Model file for the job. Use its own axes, mm. A direction names the side the tool comes from. Coordinates: 2 decimals unless noted, no trailing zeros. Write each loop counter-clockwise with the first axis right and the second up, starting at its lowest first coordinate (ties: lowest second). Pieces come first, ordered by that corner, then holes. Notation, with made-up numbers: (-11.75, -2.75) - (26.25, -2.75) arc R4 ccw to (26.25, 1.25) - close; hole circle Ø10 at (56.25, 54). An arc over 180 degrees is marked (long way). Put each result on its own line as item: value. Start each with the question number.
1. Saw through at C-C, the plane z = 0. Write the cut outline in (x, y).
2. Which spindle directions (+Z, -Z, +X, -X, +Y, -Y) get a long thin tool onto all of the face, cutting with end or side? Do faces 4 (the face through (25.19, -0.49, -25.72)), 5 (the face through (-25.19, -0.49, 25.72)), 6 (the face through (-27.15, 3.01, 20.35)). Say none if no direction does.
3. Saw through at B-B, the plane x = 0. Write the cut outline in (y, z), plus the area to 3 significant figures.
4. Pull direction Z, two halves, no side cores. Call faces 1 (the face through (27.44, 5.4, 19.86)), 2 (the face through (-1.5, -1, 35)), 3 (the face through (35, -1, -1.5)): released by +Z, released by -Z, zero draft, split by the parting line, or undercut.
5. Saw through at A-A, the plane y = 5. Write the cut outline in (x, z).
6. Drop flat-ended pins along their axis: P1, Ø1, axis at y = 3.5, z = -33, coming from the -X side; P2, Ø1.5, axis at x = -31, y = 5, coming from the +Z side; P3, Ø4, axis at x = -27, z = -6.5, coming from the +Y side. Give the stop position or say it passes through.
7. Drill centre lines: L1, parallel to X at y = -1.25, z = 6.5; L2, parallel to Y at x = -10, z = 29; L3, parallel to Z at x = -2, y = 2.5. Where is each one in solid material? Low to high. Write a range as from..to.
```python
from build123d import *

# Parameters (mm, degrees)
SKETCH1_R           = 40
BOSS_EXTRUDE1_DEPTH = 2
SKETCH2_W           = 8.4
SKETCH2_H           = 2.75
BOSS_EXTRUDE2_DEPTH = 4
SKETCH3_R           = 36
SKETCH3_R_2         = 34
BOSS_EXTRUDE3_DEPTH = 2
FILLET2_R           = 1
CUT_EXTRUDE1_DEPTH  = 2
SKETCH5_W           = 8.4
SKETCH5_H           = 2.75
SKETCH5_W_2         = 8.1
SKETCH5_H_2         = 2.45
CUT_EXTRUDE2_DEPTH  = 4
FILLET3_R           = 2


with BuildPart() as part:
    # Sketch1 → Boss-Extrude1 (new body)
    with BuildSketch(Plane(origin=(0, 0, 0), x_dir=(1, 0, 0), z_dir=(0, 1, 0))):
        with Locations(Location((0, 0, 0), (0, 0, 270))):
            Circle(SKETCH1_R)
    extrude(amount=BOSS_EXTRUDE1_DEPTH)

    # Sketch2 → Boss-Extrude2 (add)
    with BuildSketch(Plane(origin=(0, 2, 0), x_dir=(1, 0, 0), z_dir=(0, 1, 0))):
        with Locations((0, 33.675)):
            Rectangle(SKETCH2_W, SKETCH2_H)
        Polygon((32.454190403, -13.887693304), (28.254190403, -21.162306696), (25.872620542, -19.787306696), (30.072620542, -12.512693304), align=None)
        Polygon((-28.254190403, -21.162306696), (-32.454190403, -13.887693304), (-30.072620542, -12.512693304), (-25.872620542, -19.787306696), align=None)
    extrude(amount=BOSS_EXTRUDE2_DEPTH)

    # Sketch3 → Boss-Extrude3 (add)
    with BuildSketch(Plane.XZ):
        with Locations(Location((0, 0, 0), (0, 0, 90))):
            Circle(SKETCH3_R)
        with Locations(Location((0, 0, 0), (0, 0, 270))):
            Circle(SKETCH3_R_2, mode=Mode.SUBTRACT)
    extrude(amount=BOSS_EXTRUDE3_DEPTH)

    # Fillet2
    fillet2_edges = [part.edges().sort_by_distance(p)[0] for p in [
        (0, -2, -36),
        (0, -2, 34),
    ]]
    fillet(fillet2_edges, radius=FILLET2_R - 0.0001)  # a hair under: the kernel refuses the full size

    # Sketch4 → Cut-Extrude1 (cut)
    with BuildSketch(Plane.XZ):
        Polygon((-1.5, -40), (-1.5, -1.5), (-40, -1.5), (-40, 1.5), (-1.5, 1.5), (-1.5, 40), (1.5, 40), (1.5, 1.5), (40, 1.5), (40, -1.5), (1.5, -1.5), (1.5, -40), align=None)
    extrude(amount=CUT_EXTRUDE1_DEPTH, mode=Mode.SUBTRACT)

    # Sketch5 → Cut-Extrude2 (cut)
    # profile 1 of 3: a face of its own
    with BuildSketch(Plane(origin=(0, 6, 0), x_dir=(1, 0, 0), z_dir=(0, 1, 0))):
        Polygon((32.454190403, -13.887693304), (30.072620542, -12.512693304), (25.872620542, -19.787306696), (28.254190403, -21.162306696), align=None)
        Polygon((32.249286592, -13.942597115), (30.127524353, -12.717597115), (26.077524353, -19.732402885), (28.199286592, -20.957402885), align=None, mode=Mode.SUBTRACT)
    # profile 2 of 3: a face of its own
    with BuildSketch(Plane(origin=(0, 6, 0), x_dir=(1, 0, 0), z_dir=(0, 1, 0))):
        Polygon((-28.254190403, -21.162306696), (-25.872620542, -19.787306696), (-30.072620542, -12.512693304), (-32.454190403, -13.887693304), align=None)
        Polygon((-28.199286592, -20.957402885), (-26.077524353, -19.732402885), (-30.127524353, -12.717597115), (-32.249286592, -13.942597115), align=None, mode=Mode.SUBTRACT)
    # profile 3 of 3: a face of its own
    with BuildSketch(Plane(origin=(0, 6, 0), x_dir=(1, 0, 0), z_dir=(0, 1, 0))):
        with Locations((0, 33.675)):
            Rectangle(SKETCH5_W, SKETCH5_H)
        with Locations((0, 33.675)):
            Rectangle(SKETCH5_W_2, SKETCH5_H_2, mode=Mode.SUBTRACT)
    extrude(amount=-CUT_EXTRUDE2_DEPTH, mode=Mode.SUBTRACT)

    # Fillet3
    fillet3_edges = [part.edges().sort_by_distance(p)[0] for p in [
        (31.188405472, 6, 13.330097115),
        (27.138405472, 6, 20.344902885),
        (-27.138405472, 6, 20.344902885),
        (-31.188405472, 6, 13.330097115),
        (-4.05, 6, -33.675),
        (4.05, 6, -33.675),
    ]]
    fillet(fillet3_edges, radius=FILLET3_R)


solid = part.part
```
Final values:
1. outline: (-40, 0) - (40, 0) - (40, 2) - (-40, 2) - close
2. face 4: -Z, +X, -Y
2. face 5: +Z, -X, -Y
2. face 6: +Z, +Y
3. outline: (0, -40) - (2, -40) - (2, -34.9) - (6, -34.9) - (6, -32.45) - (2, -32.45) - (2, 40) - (0, 40) - close
3. area: 170 mm²
4. face 1: released by +Z
4. face 2: zero draft
4. face 3: undercut
5. outline: (-32.12, 14.17) - (-29.99, 12.95) - (-26.21, 19.5) - (-28.33, 20.73) - close; (-3.78, -34.9) - (3.78, -34.9) - (3.78, -32.45) - (-3.78, -32.45) - close; (26.21, 19.5) - (29.99, 12.95) - (32.12, 14.17) - (28.33, 20.73) - close
6. P1: stops at x = -4.05
6. P2: stops at z = 17.41
6. P3: stops at y = 2
7. L1: x = -35.38..-33.41, 33.41..35.38
7. L2: y = 0..2
7. L3: z = -34.9..-32.45
